```python
from build123d import *

# Parameters (mm, degrees)
SKETCH1_W           = 20
SKETCH1_H           = 22.5
BOSS_EXTRUDE1_DEPTH = 4
SKETCH2_R           = 2.25
CUT_EXTRUDE1_DEPTH  = 1.5
SKETCH3_R           = 3.65
CUT_EXTRUDE2_DEPTH  = 2.5
SKETCH4_W           = 4
SKETCH4_H           = 13.5
BOSS_EXTRUDE2_DEPTH = 6.5
SKETCH5_R           = 1.45
CUT_EXTRUDE3_DEPTH  = 31.797727189
FILLET1_R           = 8


with BuildPart() as part:
    # Sketch1 → Boss-Extrude1 (new body)
    with BuildSketch(Plane.XY):
        with Locations((10, -11.25)):
            Rectangle(SKETCH1_W, SKETCH1_H)
    extrude(amount=BOSS_EXTRUDE1_DEPTH)

    # Sketch2 → Cut-Extrude1 (cut)
    with BuildSketch(Plane.XY.offset(4)):
        with Locations((10, -11.25)):
            Circle(SKETCH2_R)
    extrude(amount=-CUT_EXTRUDE1_DEPTH, mode=Mode.SUBTRACT)

    # Sketch3 → Cut-Extrude2 (cut)
    with BuildSketch(Plane.XY.offset(2.5)):
        with Locations((10, -11.25)):
            Circle(SKETCH3_R)
    extrude(amount=-CUT_EXTRUDE2_DEPTH, mode=Mode.SUBTRACT)

    # Sketch4 → Boss-Extrude2 (add)
    with BuildSketch(Plane(origin=(0, 0, 0), x_dir=(-1, 0, 0), z_dir=(0, 0, -1))):
        with Locations((-18, -11.25)):
            Rectangle(SKETCH4_W, SKETCH4_H)
        Polygon((0, 0), (-20, 0), (-20, -4.5), (-16, -4.5), (-4, -4.5), (0, -4.5), align=None)
        with Locations((-2, -11.25)):
            Rectangle(SKETCH4_W, SKETCH4_H)
        Polygon((-16, -18), (-20, -18), (-20, -22.5), (0, -22.5), (0, -18), (-4, -18), align=None)
    extrude(amount=BOSS_EXTRUDE2_DEPTH)

    # Sketch5 → Cut-Extrude3 (cut, through all)
    with BuildSketch(Plane(origin=(0, 0, 0), x_dir=(1, 0, 0), z_dir=(0, 1, 0))):
        with Locations(Location((10, 1.5, 0), (0, 0, 270))):
            Circle(SKETCH5_R)
    extrude(amount=-CUT_EXTRUDE3_DEPTH, mode=Mode.SUBTRACT)

    # Fillet1
    # the kernel refuses this fillet: 8 mm, written as the material it takes off along each edge
    with BuildSketch(Plane(origin=(0, -42.5, -6.5), x_dir=(0, 0, 1), z_dir=(0, 1, 0)), Plane(origin=(20, 20, -6.5), x_dir=(0, 0, 1), z_dir=(0, -1, 0))) as fillet1_piece_1:
        with BuildLine():
            CenterArc((FILLET1_R, FILLET1_R), FILLET1_R, 180, 90)
            Line((0, FILLET1_R), (0, 0))
            Line((0, 0), (FILLET1_R, 0))
        make_face()
    extrude(amount=62.5, mode=Mode.SUBTRACT)


solid = part.part
```
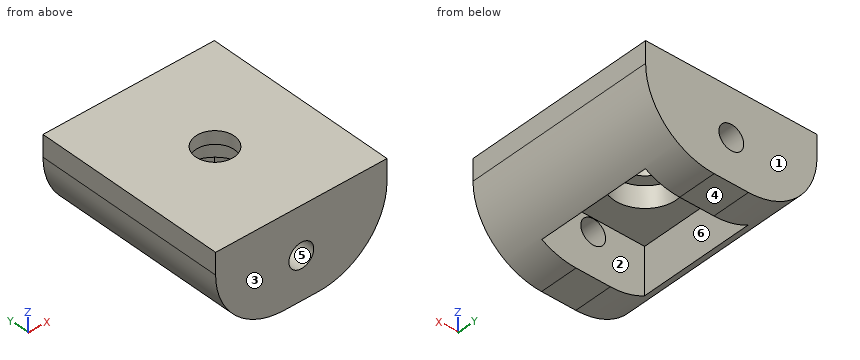
Can you work these out from the model? Positions are in its coordinate system, mm. Face numbers are marked on the shaded views. A direction names the side the tool comes from. Round coordinates to 2 decimals unless told otherwise and drop trailing zeros. Order: outer loops, then holes, each group sorted by start corner. A loop starts at its lowest first (then second) coordinate and runs counter-clockwise, first axis right, second up. Notation, with made-up numbers: (87, -21.75) -> (134, -21.75) arc R29 ccw to (134, 16.25) -> close; hole circle Ø6 at (-13, 31). An arc over 180 degrees is marked (long way). Return JSON: item names as keys, results as strings. Group by question number.
1. If we section it at B-B, the plane x = 10: Write out the boundary of the cut face in (y, z), then the cut area to 3 significant figures.
2. I need wall thicknesses on line 1 (Y direction, x = 10, z = 1.5); line 2 (Y direction, x = 8.25, z = -3); line 3 (X direction, y = -1.9, z = -1.5). Which ranges of each line are inside material? Lowest first, please. Write a range as [from, to].
3. Will these pins go through, and if not, where does the flat tip stop? pin 1 (3.5 mm diameter, centred on x = 9, y = -12, fed in from -Z); pin 2 (1.6 mm diameter, centred on y = -10.5, z = -3, fed in from -X); pin 3 (1 mm diameter, centred on y = -5.5, z = -0.5, fed in from -X).
4. If we section it at D-D, the plane z = -1.5: Write out the boundary of the cut face in (x, y).
5. We'd pull the mould along Y, two halves only. Please class the marked faces 1, 2, 3 and 4: released by +Y, released by -Y, zero draft, split by the parting line, or undercut.
6. If we section it at A-A, the plane y = -11.25: Write out the boundary of the cut face in (x, z), then the cut area to 3 significant figures.
7. If we section it at C-C, the plane y = -7: Write out the boundary of the cut face in (x, z).
8. Which directions (+Z, -Z, +X, -X, +Y, -Y) give clear straight access to the entire face, cutting with the end or side of a thin tool? Please do the marked faces 5 and 6.
Output values:
{
 "1": {"outline": "(-22.5, -6.5) -> (-18, -6.5) -> (-18, -2.95) -> (-22.5, -2.95) -> close; (-22.5, -0.05) -> (-18, -0.05) -> (-18, 0) -> (-14.9, 0) -> (-14.9, 2.5) -> (-13.5, 2.5) -> (-13.5, 4) -> (-22.5, 4) -> close; (-9, 2.5) -> (-7.6, 2.5) -> (-7.6, 0) -> (-4.5, 0) -> (-4.5, -0.05) -> (0, -0.05) -> (0, 4) -> (-9, 4) -> close; (-4.5, -6.5) -> (0, -6.5) -> (0, -2.95) -> (-4.5, -2.95) -> close", "area": "97.4 mm²"},
 "2": {"line 1": "[-22.5, -14.9], [-7.6, 0]", "line 2": "[-22.5, -18], [-4.5, 0]", "line 3": "[0.58, 8.55], [11.45, 19.42]"},
 "3": {"pin 1": "z = 2.5", "pin 2": "x = 0.91", "pin 3": "x = 0.14"},
 "4": {"outline": "(0.58, -22.5) -> (8.55, -22.5) -> (8.55, -18) -> (4, -18) -> (4, -4.5) -> (8.55, -4.5) -> (8.55, 0) -> (0.58, 0) -> close; (11.45, -22.5) -> (19.42, -22.5) -> (19.42, 0) -> (11.45, 0) -> (11.45, -4.5) -> (16, -4.5) -> (16, -18) -> (11.45, -18) -> close"},
 "5": {"face 1": "released by +Y", "face 2": "undercut", "face 3": "released by -Y", "face 4": "zero draft"},
 "6": {"outline": "(0, 1.5) arc R8 ccw to (4, -5.43) -> (4, 0) -> (6.35, 0) -> (6.35, 2.5) -> (7.75, 2.5) -> (7.75, 4) -> (0, 4) -> close; (12.25, 2.5) -> (13.65, 2.5) -> (13.65, 0) -> (16, 0) -> (16, -5.43) arc R8 ccw to (20, 1.5) -> (20, 4) -> (12.25, 4) -> close", "area": "82.3 mm²"},
 "7": {"outline": "(0, 1.5) arc R8 ccw to (4, -5.43) -> (4, 0) -> (16, 0) -> (16, -5.43) arc R8 ccw to (20, 1.5) -> (20, 4) -> (0, 4) -> close"},
 "8": {"face 5": "+Y, -Y", "face 6": "-Z"}
}
